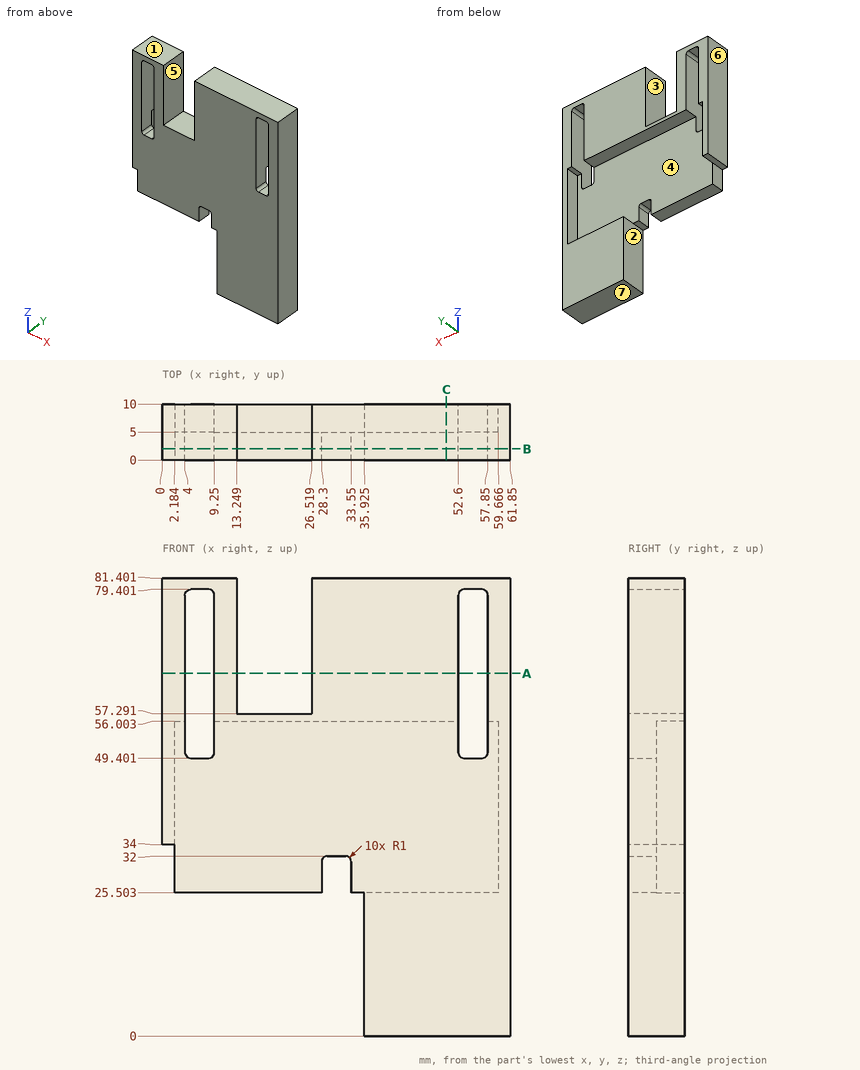
Can you work these out from the drawing? Everything is in mm from the part's minimum corner. A direction names the side the tool comes from. Give positions to 0.01 mm unless a question says otherwise; leave off trailing zeros. Order: outer loops, then holes, each group sorted by start corner. A loop starts at its lowest first (then second) coordinate and runs counter-clockwise, first axis right, second up. Notation, with made-up numbers: M 70.5,12 L 98.5,12 A12 ccw 98.5,17 Z; hole C 40.25,39 d6. An arc over 180 degrees is marked long. Use a Markdown table: item, result. Add a question column.
1. Suppose I cut it at A-A (z = 64.5). List the corners of the cut face in (x, y) for me.
2. On a 3-axis mill with a long thin cutter (end or side, diameter ignored), from which of +Z, -Z, +X, -X, +Y, -Y can I reach the whole of each face in a straight line? I mean the marked faces 1, 2 and 3. Say none if no direction works.
3. Suppose I cut it at B-B (y = 2). Give the number of separate pieces and of enclosed holes in the cut face, and give its area (3 significant figures).
4. For pin 1 Ø4 at (y, z) = (3.5, 30) entering from -X; pin 2 Ø4 at (x, y) = (21, 3.5) entering from -Z; pin 3 Ø10 at (x, z) = (17, 40) entering from +Y; pin 4 Ø2.5 at (x, y) = (54.5, 6.5) entering from -Z, each with a flat end and sliding along its axis, tell me the tip position at first contact or that it passes through.
5. Suppose I cut it at C-C (x = 50.5). List the corners of the cut face in (y, z) for me.
6. If we mould it in two halves opening along X, with no side actions, what happens to the marked faces 4, 5, 6 and 7? For each: +X half, -X half, draft (parallel to the pull), parting line (faces both ways), or undercut.
7. I need wall thicknesses on probe 1 along X at (y, z) = (9, 76.5); probe 2 along Z at (x, y) = (44.5, 9.25); probe 3 along Z at (x, y) = (57, 9). Which ranges of each line are inside material? Lowest first, please. Write a range as from..to.
Results list:
| question | item | result |
|---|---|---|
| 1 | outline | M 0,0 L 4,0 L 4,10 L 0,10 Z; M 9.25,0 L 13.25,0 L 13.25,10 L 9.25,10 Z; M 26.52,0 L 52.6,0 L 52.6,10 L 26.52,10 Z; M 57.85,0 L 61.85,0 L 61.85,10 L 57.85,10 Z |
| 2 | face 1 | +Z, +X, -X, +Y, -Y |
| 2 | face 2 | -Z, -X, +Y, -Y |
| 2 | face 3 | +Z, +Y, -Y |
| 3 | separate pieces | 1 |
| 3 | enclosed holes | 2 |
| 3 | area | 3,430 mm² |
| 4 | pin 1 | stops at x = 2.18 |
| 4 | pin 2 | stops at z = 25.5 |
| 4 | pin 3 | stops at y = 5 |
| 4 | pin 4 | stops at z = 0 |
| 5 | outline | M 0,0 L 10,0 L 10,25.5 L 5,25.5 L 5,56 L 10,56 L 10,81.4 L 0,81.4 Z |
| 6 | face 4 | undercut |
| 6 | face 5 | undercut |
| 6 | face 6 | -X half |
| 6 | face 7 | draft |
| 7 | probe 1 | x = 0..4, 9.25..13.25, 26.52..52.6, 57.85..61.85 |
| 7 | probe 2 | z = 0..25.5, 56..81.4 |
| 7 | probe 3 | z = 0..25.5, 79.39..81.4 |
